from build123d import *

# Parameters (mm, degrees)
SKETCH_1_W               = 8
SKETCH_1_H               = 8
SKETCH_1_W_2             = 4
SKETCH_1_H_2             = 4
EXTRUDE_1_DEPTH          = 205
SKETCH_7_R               = 6
EXTRUDE_2_DEPTH          = 205
CUT_EXTRUDE_1_DEPTH      = 206.175534604
CUT_EXTRUDE_1_DEPTH_BACK = 206.175534604
SKETCH_2_R               = 1.65
CUT_EXTRUDE_2_DEPTH      = 206.17553471
CUT_EXTRUDE_2_DEPTH_BACK = 206.17553471
SKETCH_3_R               = 1.65
CUT_EXTRUDE_3_DEPTH      = 206.17553471
CUT_EXTRUDE_3_DEPTH_BACK = 206.17553471
SKETCH_4_R               = 1.65
CUT_EXTRUDE_4_DEPTH      = 206.17553471
CUT_EXTRUDE_4_DEPTH_BACK = 206.17553471
SKETCH_5_R               = 1.65


with BuildPart() as part:
    # 草图1 → 凸台-拉伸1 (new body)
    with BuildSketch(Plane.XY):
        Rectangle(SKETCH_1_W, SKETCH_1_H)
        Rectangle(SKETCH_1_W_2, SKETCH_1_H_2, mode=Mode.SUBTRACT)
    extrude(amount=EXTRUDE_1_DEPTH)

    # 草图7 → 凸台-拉伸2 (add)
    with BuildSketch(Plane(origin=(0, 0, 0), x_dir=(-1, 0, 0), z_dir=(0, 0, -1))):
        Circle(SKETCH_7_R)
    extrude(amount=-EXTRUDE_2_DEPTH)

    # 草图2 → 切除-拉伸1 (cut, two sides: drawn at the far end of the back side and taken through both)
    with BuildSketch(Plane(origin=(0, 0, 0), x_dir=(1, 0, 0), z_dir=(0, 1, 0)).offset(-CUT_EXTRUDE_1_DEPTH_BACK)):
        with Locations(Location((0, -5, 0), (0, 0, 270))):
            Circle(SKETCH_2_R)
        with Locations(Location((0, -15, 0), (0, 0, 270))):
            Circle(SKETCH_2_R)
    extrude(amount=CUT_EXTRUDE_1_DEPTH + CUT_EXTRUDE_1_DEPTH_BACK, mode=Mode.SUBTRACT)

    # 草图3 → 切除-拉伸2 (cut, two sides: drawn at the far end of the back side and taken through both)
    with BuildSketch(Plane.ZY.offset(-CUT_EXTRUDE_2_DEPTH_BACK)):
        with Locations((10, 0)):
            Circle(SKETCH_3_R)
        with Locations((20, 0)):
            Circle(SKETCH_3_R)
    extrude(amount=CUT_EXTRUDE_2_DEPTH + CUT_EXTRUDE_2_DEPTH_BACK, mode=Mode.SUBTRACT)

    # 草图4 → 切除-拉伸3 (cut, two sides: drawn at the far end of the back side and taken through both)
    with BuildSketch(Plane.ZY.offset(-CUT_EXTRUDE_3_DEPTH_BACK)):
        with Locations((200, 0)):
            Circle(SKETCH_4_R)
        with Locations((185, 0)):
            Circle(SKETCH_4_R)
    extrude(amount=CUT_EXTRUDE_3_DEPTH + CUT_EXTRUDE_3_DEPTH_BACK, mode=Mode.SUBTRACT)

    # 草图5 → 切除-拉伸4 (cut, two sides: drawn at the far end of the back side and taken through both)
    with BuildSketch(Plane(origin=(0, 0, 0), x_dir=(1, 0, 0), z_dir=(0, 1, 0)).offset(-CUT_EXTRUDE_4_DEPTH_BACK)):
        with Locations(Location((0, -190, 0), (0, 0, 270))):
            Circle(SKETCH_5_R)
        with Locations(Location((0, -175, 0), (0, 0, 270))):
            Circle(SKETCH_5_R)
    extrude(amount=CUT_EXTRUDE_4_DEPTH + CUT_EXTRUDE_4_DEPTH_BACK, mode=Mode.SUBTRACT)


solid = part.part
Work out the finished part from the listing and answer in its coordinate system (mm). Give positions to 0.01 mm unless a question says otherwise; leave off trailing zeros. Order: outer loops, then holes, each group sorted by start corner. A loop starts at its lowest first (then second) coordinate and runs counter-clockwise, first axis right, second up. Notation, with made-up numbers: (47, -12.75) - (52, -12.75) arc R35 ccw to (52, 26.25) - close; hole circle Ø7 at (76, 45). An arc over 180 degrees is marked (long way). Answer as CSV lines item,"result". Start each with the question number.
Q1. The part is cut by section A-A (x = 0). Give the number of separate pieces and of enclosed holes in the cut face, then the cut area to 3 significant figures.
Q2. The mould has two halves that part along Y. Classify faces 1 (the face through (0.084, 0.496, 201.574)), 2 (the face through (0.08, -1, 18.69)), 3 (the face through (0, 0, 205)), 4 (the face through (-5.723, 1.802, 101.065)): +Y half, -Y half, draft (parallel to the pull), parting line (faces both ways), or undercut.
Q3. Find the intervals of material crossed by L1, parallel to Z at x = -1.75, y = 0; L2, parallel to Z at x = 4.5, y = -1; L3, parallel to Y at x = 1, z = 200, in increasing order. Write a range as [from, to].
Q4. The part is cut by section B-B (y = 4). Write down the section's boundary in (x, z), then the cut area to 3 significant figures.
Q5. The part is cut by section C-C (z = 15). Write down the section's boundary in (x, y).
Q6. The part is cut by section D-D (z = 144). Write down the section's boundary in (x, y).
Q7. Given pin 1 Ø1.5 at (y, z) = (4.5, 99.5) entering from +X; pin 2 Ø1 at (y, z) = (-4, 23) entering from +X; pin 3 Ø2 at (y, z) = (-3.5, 33) entering from +X, each flat-ended and moving along its own axis, determine where each tip first touches the part or whether it passes through.
Check result:
1,separate pieces,"5"
1,enclosed holes,"4"
1,area,"2,270 mm²"
2,face 1,"undercut"
2,face 2,"undercut"
2,face 3,"draft"
2,face 4,"parting line"
3,L1,"z = [0, 8.35], [11.65, 18.35], [21.65, 183.35], [186.65, 198.35], [201.65, 205]"
3,L2,"z = [0, 8.69], [11.31, 18.69], [21.31, 183.69], [186.31, 198.69], [201.31, 205]"
3,L3,"y = [-5.92, -1.65], [1.65, 5.92]"
4,outline,"(-4.47, 0) - (4.47, 0) - (4.47, 205) - (-4.47, 205) - close; hole circle Ø3.3 at (0, 5); hole circle Ø3.3 at (0, 15); hole circle Ø3.3 at (0, 175); hole circle Ø3.3 at (0, 190)"
4,area,"1,800 mm²"
5,outline,"(-1.65, -5.77) - (-1.65, 5.77) arc R6 ccw to start; (1.65, -5.77) arc R6 ccw to (1.65, 5.77) - close"
6,outline,"circle Ø12 at (0, 0)"
7,pin 1,"stops at x = 4.68"
7,pin 2,"stops at x = 4.87"
7,pin 3,"stops at x = 5.45"
